```python
from build123d import *

# Parameters (mm, degrees)
F0_W     = 127
F0_H     = 127
F0_R     = 12.7
F1_DEPTH = 127
F2_W     = 38.1
F2_H     = 63.5
F3_DEPTH = 25.4
F4_W     = 38.1
F4_H     = 31.75
F5_DEPTH = 76.2


with BuildPart() as f1:
    # F0 (on Front) → F1 (new body)
    with BuildSketch(Plane.XZ):
        Rectangle(F0_W, F0_H)
        with Locations((-31.75, -31.75)):
            Circle(F0_R, mode=Mode.SUBTRACT)
        with Locations((31.75, -31.75)):
            Circle(F0_R, mode=Mode.SUBTRACT)
        with Locations((-31.75, 31.75)):
            Circle(F0_R, mode=Mode.SUBTRACT)
        with Locations((31.75, 31.75)):
            Circle(F0_R, mode=Mode.SUBTRACT)
    extrude(amount=F1_DEPTH)

    # F2 (on face) → F3 (cut)
    with BuildSketch(Plane.YZ.offset(63.5)):
        with Locations((-63.5, 31.75)):
            Rectangle(F2_W, F2_H)
    extrude(amount=-F3_DEPTH, mode=Mode.SUBTRACT)

    # F4 (on face) → F5 (cut)
    with BuildSketch(Plane.YZ.offset(38.1)):
        with Locations((-63.5, 47.625)):
            Rectangle(F4_W, F4_H)
    extrude(amount=-F5_DEPTH, mode=Mode.SUBTRACT)


solid = f1.part
```
Geometry: final body of the model. Coordinates: model frame, mm. A direction names the side the tool comes from. Coordinates: 2 decimals unless noted, no trailing zeros. Write each loop counter-clockwise with the first axis right and the second up, starting at its lowest first coordinate (ties: lowest second). Pieces come first, ordered by that corner, then holes. Notation, with made-up numbers: M -35,-16 L -3,-16 A8 ccw -3,-7 Z; hole C -3,89 d3. An arc over 180 degrees is marked long. Use CSV: the item, a comma, the result in double quotes. Start each with the question number.
1. Cut plane D-D on x = 15.5. Return the cut outline in (y, z), plus the area to 3 significant figures.
2. Cut plane C-C on y = -115. Return the cut outline in (x, z), plus the area to 3 significant figures.
3. Mould query, pull axis X, two halves, no side actions, for faces 3 (the face through (-1, -91, 63.5)), 4 (the face through (-41.828, -62.611, 24.022)), 5 (the face through (38.1, -64, 11)). Classes: pulls with the +X half, pulls with the -X half, needs draft (parallel to the pull), parting line crosses it, or undercut.
4. Cut plane A-A on z = -31.75. Return the cut outline in (x, y).
5. Ray query, probe 1 along Z at (x, y) = (-31.75, -36); probe 2 along X at (y, z) = (-96, 31); probe 3 along Y at (x, z) = (-12, 36.5). Return the intervals inside material, ascending.
6. Cut plane B-B on x = -31.75. Return the cut outline in (y, z).
7. Reachability of faces 1 (the face through (63.5, -63, -1)), 2 (the face through (25, -82.55, 45)) from +Z, -Z, +X, -X, +Y, -Y: full face, straight path, thin tool, end or side. Return the list, or none.
8. First-contact query: P1, Ø23, axis at y = -69.5, z = 57.5, coming from the +X side; P2, Ø20.5, axis at x = 54.5, y = -61, coming from the +Z side; P3, Ø16.5, axis at y = -62.5, z = 9, coming from the +X side; P4, Ø15, axis at x = 31.75, z = 31.75, coming from the +Y side. Flat tips, straight axial feed; report the tip coordinate or a pass-through.
Entries:
1,outline,"M -127,-63.5 L 0,-63.5 L 0,63.5 L -44.45,63.5 L -44.45,31.75 L -82.55,31.75 L -82.55,63.5 L -127,63.5 Z"
1,area,"14,900 mm²"
2,outline,"M -63.5,-63.5 L 63.5,-63.5 L 63.5,63.5 L -63.5,63.5 Z; hole C -31.75,-31.75 d25.4; hole C -31.75,31.75 d25.4; hole C 31.75,-31.75 d25.4; hole C 31.75,31.75 d25.4"
2,area,"14,100 mm²"
3,face 3,"needs draft"
3,face 4,"undercut"
3,face 5,"pulls with the +X half"
4,outline,"M -63.5,-127 L -44.45,-127 L -44.45,0 L -63.5,0 Z; M -19.05,-127 L 19.05,-127 L 19.05,0 L -19.05,0 Z; M 44.45,-127 L 63.5,-127 L 63.5,0 L 44.45,0 Z"
5,probe 1,"-63.5 to -44.45, -19.05 to 19.05, 44.45 to 63.5"
5,probe 2,"-63.5 to -44.43, -19.07 to 19.07, 44.43 to 63.5"
5,probe 3,"-127 to -82.55, -44.45 to 0"
6,outline,"M -127,-63.5 L 0,-63.5 L 0,-44.45 L -127,-44.45 Z; M -127,-19.05 L 0,-19.05 L 0,19.05 L -127,19.05 Z; M -127,44.45 L -82.55,44.45 L -82.55,63.5 L -127,63.5 Z; M -44.45,44.45 L 0,44.45 L 0,63.5 L -44.45,63.5 Z"
7,face 1,"+Z, -Z, +X, +Y, -Y"
7,face 2,"+Z, +X"
8,P1,"x = -38.1"
8,P2,"z = 0"
8,P3,"x = 38.1"
8,P4,"through"
